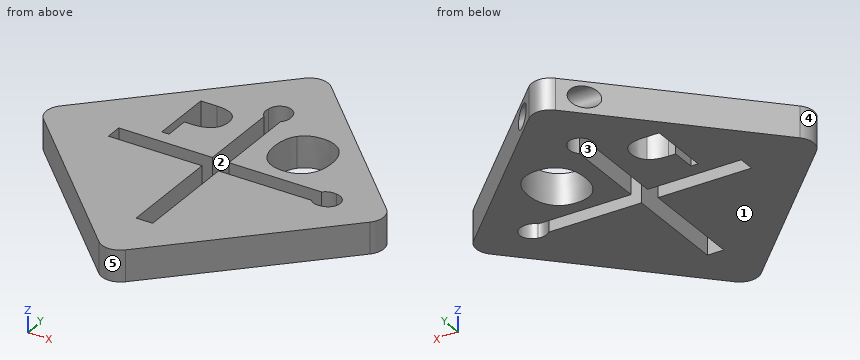
```python
from build123d import *

# Parameters (mm, degrees)
F1_DEPTH = 2.5
F2_R     = 0.85
F3_DEPTH = 12.5


with BuildPart() as f1:
    # F0 (on Top) → F1 (new body)
    with BuildSketch(Plane.XY):
        with BuildLine():
            Line((13.081475452, -13.081475452), (1.0606601718, -1.0606601718))
            ThreePointArc((1.0606601718, -1.0606601718), (0, -0.6213203436), (-1.0606601718, -1.0606601718))
            Line((-1.0606601718, -1.0606601718), (-13.081475452, -13.081475452))
            ThreePointArc((-13.081475452, -13.081475452), (-13.5208152802, -14.1421356237), (-13.081475452, -15.2027957955))
            Line((-13.081475452, -15.2027957955), (-1.0606601718, -27.2236110757))
            ThreePointArc((-1.0606601718, -27.2236110757), (0, -27.6629509039), (1.0606601718, -27.2236110757))
            Line((1.0606601718, -27.2236110757), (13.081475452, -15.2027957955))
            ThreePointArc((13.081475452, -15.2027957955), (13.5208152802, -14.1421356237), (13.081475452, -13.081475452))
        make_face()
        with BuildLine():
            add(Edge.make_bspline(
                [(-4.0900345447, -7.4211291907), (-2.2323956558, -7.4211291907), (-2.2323956558, -8.8653566212)],
                knots=[0, 0, 0, 1, 1, 1], degree=2))
            add(Edge.make_bspline(
                [(-2.2323956558, -8.8653566212), (-2.2323956558, -9.6183948157), (-2.7461760377, -10.0236682532)],
                knots=[0, 0, 0, 1, 1, 1], degree=2))
            add(Edge.make_bspline(
                [(-2.7461760377, -10.0236682532), (-3.2599564197, -10.4289416907), (-4.2159026002, -10.4289416907)],
                knots=[0, 0, 0, 1, 1, 1], degree=2))
            Line((-4.2159026002, -10.4289416907), (-4.7996699613, -10.4289416907))
            Line((-4.7996699613, -10.4289416907), (-4.7996699613, -12.3788114823))
            Line((-4.7996699613, -12.3788114823), (-5.3758418363, -12.3788114823))
            Line((-5.3758418363, -12.3788114823), (-5.3758418363, -7.4211291907))
            Line((-5.3758418363, -7.4211291907), (-4.0900345447, -7.4211291907))
        make_face(mode=Mode.SUBTRACT)
        with BuildLine():
            Line((-8.1334756687, -14.8039748892), (-8.1334756687, -13.4802963582))
            Line((-8.1334756687, -13.4802963582), (-0.6236797201, -13.4802963582))
            Line((-0.6236797201, -13.4802963582), (-0.6236797201, -6.9198086858))
            ThreePointArc((-0.6236797201, -6.9198086858), (-0.9032194318, -6.4583786209), (-0.9135835525, -5.9189782686))
            ThreePointArc((-0.9135835525, -5.9189782686), (0.0168397474, -5.0141534426), (0.9868078824, -5.876451129))
            ThreePointArc((0.9868078824, -5.876451129), (0.9900106564, -6.4384308628), (0.6999988109, -6.9198086858))
            Line((0.6999988109, -6.9198086858), (0.6999988109, -13.4802963582))
            Line((0.6999988109, -13.4802963582), (8.1334756687, -13.4802963582))
            ThreePointArc((8.1334756687, -13.4802963582), (8.5949057336, -13.2007566465), (9.134306086, -13.1903925258))
            ThreePointArc((9.134306086, -13.1903925258), (10.0391309119, -14.1208158258), (9.1768332255, -15.0907839607))
            ThreePointArc((9.1768332255, -15.0907839607), (8.6148534917, -15.0939867347), (8.1334756687, -14.8039748892))
            Line((8.1334756687, -14.8039748892), (0.6999988109, -14.8039748892))
            Line((0.6999988109, -14.8039748892), (0.6999988109, -23.1867600232))
            Line((0.6999988109, -23.1867600232), (-0.6236797201, -23.1867600232))
            Line((-0.6236797201, -23.1867600232), (-0.6236797201, -14.8039748892))
            Line((-0.6236797201, -14.8039748892), (-8.1334756687, -14.8039748892))
        make_face(mode=Mode.SUBTRACT)
        with BuildLine():
            add(Edge.make_bspline(
                [(6.0662657395, -8.0211739904), (6.6663091423, -8.6993423932), (6.6663091423, -9.8929187821)],
                knots=[0, 0, 0, 1, 1, 1], degree=2))
            add(Edge.make_bspline(
                [(6.6663091423, -9.8929187821), (6.6663091423, -11.0832399627), (6.0640956006, -11.7652061085)],
                knots=[0, 0, 0, 1, 1, 1], degree=2))
            add(Edge.make_bspline(
                [(6.0640956006, -11.7652061085), (5.4618820589, -12.4471722543), (4.3909185173, -12.4471722543)],
                knots=[0, 0, 0, 1, 1, 1], degree=2))
            add(Edge.make_bspline(
                [(4.3909185173, -12.4471722543), (3.2960834478, -12.4471722543), (2.7009228576, -11.7771418724)],
                knots=[0, 0, 0, 1, 1, 1], degree=2))
            add(Edge.make_bspline(
                [(2.7009228576, -11.7771418724), (2.1057622673, -11.1071114904), (2.1057622673, -9.8864083654)],
                knots=[0, 0, 0, 1, 1, 1], degree=2))
            add(Edge.make_bspline(
                [(2.1057622673, -9.8864083654), (2.1057622673, -8.6754708654), (2.7025504617, -8.0092382265)],
                knots=[0, 0, 0, 1, 1, 1], degree=2))
            add(Edge.make_bspline(
                [(2.7025504617, -8.0092382265), (3.2993386562, -7.3430055877), (4.3974289339, -7.3430055877)],
                knots=[0, 0, 0, 1, 1, 1], degree=2))
            add(Edge.make_bspline(
                [(4.3974289339, -7.3430055877), (5.4662223367, -7.3430055877), (6.0662657395, -8.0211739904)],
                knots=[0, 0, 0, 1, 1, 1], degree=2))
        make_face(mode=Mode.SUBTRACT)
    extrude(amount=F1_DEPTH)

    # F2 (on Right) → F3 (cut, symmetric)
    with BuildSketch(Plane.YZ):
        with Locations((-2.4908210296, 1.292226194)):
            Circle(F2_R)
    extrude(amount=F3_DEPTH, both=True, mode=Mode.SUBTRACT)


solid = f1.part
```
CAD build for the part. Positions are in the model's coordinates, mm. Face numbers are marked on the shaded views. A direction names the side the tool comes from. Round coordinates to 2 decimals unless told otherwise and drop trailing zeros. Order: outer loops, then holes, each group sorted by start corner. A loop starts at its lowest first (then second) coordinate and runs counter-clockwise, first axis right, second up. Notation, with made-up numbers: (-15.5, 82) - (-1.5, 82) arc R19 ccw to (-1.5, 94) - close; hole circle Ø2 at (40.5, -3). An arc over 180 degrees is marked (long way). Answer as CSV lines item,"result". Start each with the question number.
1. Saw through at C-C, the plane y = -4. Write the cut outline in (x, z).
2. Pin check, flat tips, straight feed: pin 1 (1 mm diameter, centred on x = -4.5, z = 1.5, fed in from -Y); pin 2 (0.5 mm diameter, centred on x = -5, z = 1.5, fed in from +Y); pin 3 (0.8 mm diameter, centred on x = -6, z = 1, fed in from +Y). Stop position of each tip, or through.
3. Saw through at A-A, the plane y = -19. Write the cut outline in (x, z).
4. Saw through at D-D, the plane x = 11.25. Write the cut outline in (y, z), and give its area (3 significant figures).
5. Tool access for the marked faces 1 and 2: list every direction of +Z, -Z, +X, -X, +Y, -Y with a clear straight run to the whole face (end or side of a thin tool).
6. Saw through at B-B, the plane z = 0.8. Count the separate pieces of the cut face and the enclosed holes in it, and give its area (3 significant figures).
7. Drill centre lines: L1, parallel to Z at x = -1, y = -2.5; L2, parallel to Y at x = 5, z = 0.5; L3, parallel to Y at x = 5.5, z = 1.1. Where is each one in solid material? Low to high. Write a range as [from, to].
8. Pull direction X, two halves, no side cores. Call the marked faces 3, 4 and 5: +X half, -X half, draft (parallel to the pull), parting line (faces both ways), or undercut.
Model answer:
1,outline,"(-4, 0) - (4, 0) - (4, 2.5) - (-4, 2.5) - close"
2,pin 1,"stops at y = -24.28"
2,pin 2,"stops at y = -4.75"
2,pin 3,"stops at y = -5.6"
3,outline,"(-9.28, 0) - (-0.62, 0) - (-0.62, 2.5) - (-9.28, 2.5) - close; (0.7, 0) - (9.28, 0) - (9.28, 2.5) - (0.7, 2.5) - close"
4,outline,"(-17.03, 0) - (-11.25, 0) - (-11.25, 2.5) - (-17.03, 2.5) - close"
4,area,"14.5 mm²"
5,face 1,"-Z, +X, -X, +Y, -Y"
5,face 2,"+Z, -Z"
6,separate pieces,"2"
6,enclosed holes,"3"
6,area,"315 mm²"
7,L1,"z = [0, 0.44], [2.14, 2.5]"
7,L2,"y = [-23.28, -14.8], [-13.48, -12.38], [-7.4, -5]"
7,L3,"y = [-22.78, -14.8], [-13.48, -12.21], [-7.58, -5.5]"
8,face 3,"undercut"
8,face 4,"-X half"
8,face 5,"parting line"
